Check sheet for the drawn part. Datum: minimum x, y, z corner. Units: mm. Give positions to 0.01 mm unless a question says otherwise; leave off trailing zeros. Write each loop counter-clockwise with the first axis right and the second up, starting at its lowest first coordinate (ties: lowest second). Pieces come first, ordered by that corner, then holes.
(1) Cross-section at C-C (z = 0.4). Record the boundary of the cut face in (x, y), and give its area (3 significant figures).
(2) Cross-section at A-A (y = 17). Record the boundary of the cut face in (x, z).
(3) Cross-section at D-D (y = 5.5). Record the boundary of the cut face in (x, z), and give its area (3 significant figures).
(4) Thickness scan on line 1 along X through (y, z) = (17, 1.45); line 2 along Y through (x, z) = (27.5, 1.25); line 3 along X through (y, z) = (14.5, 1). Record the ranges inside material, lowest first.
(5) Cross-section at B-B (x = 27.5). Record the boundary of the cut face in (y, z), and give its area (3 significant figures).
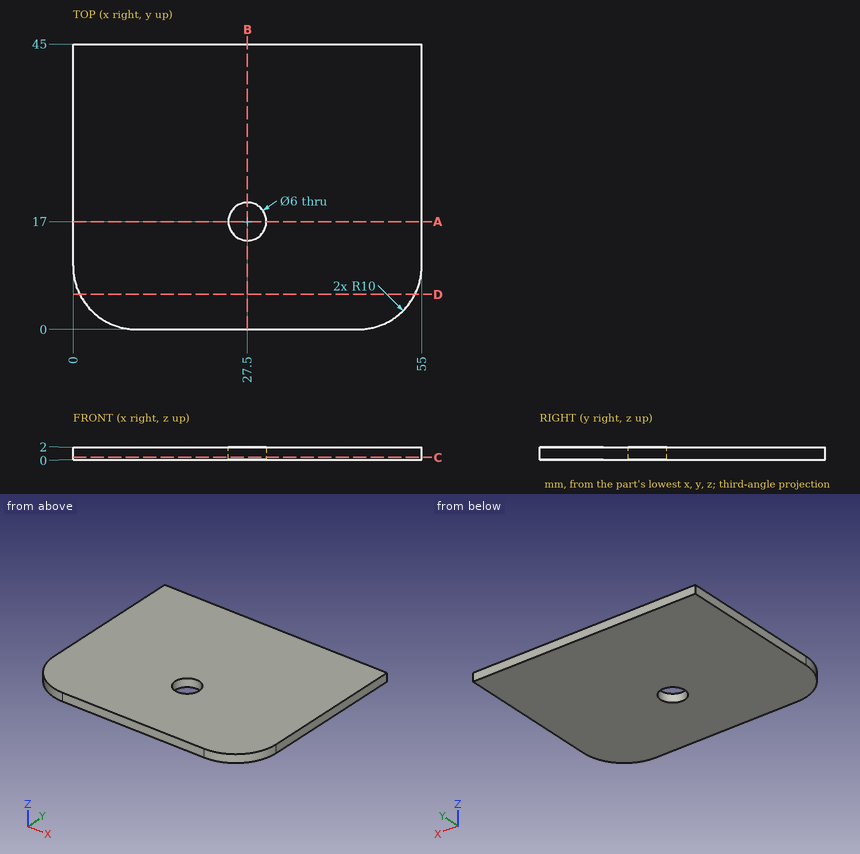
Reply:
1. outline: (0, 10) arc R10 ccw to (10, 0) - (45, 0) arc R10 ccw to (55, 10) - (55, 45) - (0, 45) - close; hole circle Ø6 at (27.5, 17)
1. area: 2,400 mm2
2. outline: (0, 0) - (24.5, 0) - (24.5, 2) - (0, 2) - close; (30.5, 0) - (55, 0) - (55, 2) - (30.5, 2) - close
3. outline: (1.07, 0) - (53.93, 0) - (53.93, 2) - (1.07, 2) - close
3. area: 106 mm2
4. line 1: x = 0 to 24.5, 30.5 to 55
4. line 2: y = 0 to 14, 20 to 45
4. line 3: x = 0 to 25.84, 29.16 to 55
5. outline: (0, 0) - (14, 0) - (14, 2) - (0, 2) - close; (20, 0) - (45, 0) - (45, 2) - (20, 2) - close
5. area: 78.0 mm2
